Autodesk Inventor part; units mm, degrees
ref_plane "YZ Plane" through (0, 0, 0) normal (1, 0, 0) x (0, 1, 0)
ref_plane "XZ Plane" through (0, 0, 0) normal (0, 1, 0) x (-1, 0, 0)
ref_plane "XY Plane" through (0, 0, 0) normal (0, 0, 1) x (1, 0, 0)
ref_plane "Work Plane1" through (0, 0, 0) normal (0, 0, 1) x (1, 0, 0)
sketch "Sketch1" plane through (0, 0, 0) normal (0, 0, 1) x (1, 0, 0)
  circle A0 centre (0, 0) radius 3.0861
  circle A1 centre (6.35, 0) radius 1.5875
  circle A2 centre (0, 6.35) radius 1.5875
  circle A3 centre (-6.35, 0) radius 1.5875
  circle A4 centre (0, -6.35) radius 1.5875
  circle A5 centre (0, 0) radius 19.2656
  point P0 (0, 0)
extrude "Extrusion1" add sketch "Sketch1" along normal blind 6.35
properties part number "smallGearMag01"
Design review of the part built by this model. Coordinates are the model's own, in mm. Give positions to 0.01 mm unless a question says otherwise; leave off trailing zeros. Loops run counter-clockwise (first coordinate to the right, second up) from the corner with the lowest first, then second, coordinate; pieces in that order, holes last. Notation, with made-up numbers: (10, 7) - (20, 7) arc R21 cw to (20, 13) - close; hole circle Ø1 at (-23, 29.5). An arc over 180 degrees is marked (long way). Write item = value, one per line.
1) Take a section at C-C on x = -5.5. State the section outline as (y, z) points.
Result sheet:
outline = (-18.46, 0) - (-1.34, 0) - (-1.34, 6.35) - (-18.46, 6.35) - close; (1.34, 0) - (18.46, 0) - (18.46, 6.35) - (1.34, 6.35) - close
2) Clearance check with flat-ended pins moving along their axes: pin 1 Ø5 at (x, y) = (6.35, 0) entering from -Z; pin 2 Ø1.9 at (x, y) = (0, -6.35) entering from +Z; pin 3 Ø1.5 at (x, z) = (-7, 2) entering from -Y; pin 4 Ø3 at (y, z) = (-10.5, 1.5) entering from +X. State where each tip first meets the part, or that it passes through.
Result sheet:
pin_1 = 0
pin_2 = through
pin_3 = -18.22
pin_4 = 17.03
3) Take a section at A-A on x = 0. State the section outline as (y, z) points, and give its area (3 significant figures).
Result sheet:
outline = (-19.27, 0) - (-7.94, 0) - (-7.94, 6.35) - (-19.27, 6.35) - close; (-4.76, 0) - (-3.09, 0) - (-3.09, 6.35) - (-4.76, 6.35) - close; (3.09, 0) - (4.76, 0) - (4.76, 6.35) - (3.09, 6.35) - close; (7.94, 0) - (19.27, 0) - (19.27, 6.35) - (7.94, 6.35) - close
area = 165 mm2
4) Take a section at D-D on z = 2.5. Count the separate pieces of the cut face and the enclosed holes in it, and give its area (3 significant figures).
Result sheet:
separate_pieces = 1
enclosed_holes = 5
area = 1,100 mm2
5) To check wall thickness, follow line 1 (Y direction, x = 0, z = 4.5); line 2 (Y direction, x = 1, z = 2.75); line 3 (X direction, y = 2, z = 1.25). State the ranges of each line that lie inside material, in increasing order.
Result sheet:
line_1 = -19.27 to -7.94, -4.76 to -3.09, 3.09 to 4.76, 7.94 to 19.27
line_2 = -19.24 to -7.58, -5.12 to -2.92, 2.92 to 5.12, 7.58 to 19.24
line_3 = -19.16 to -2.35, 2.35 to 19.16
